Source: CAD feature listing. Evaluate the final solid. Frame: model axes, mm. A direction names the side the tool comes from. Coordinates: 2 decimals unless noted, no trailing zeros. Order: outer loops, then holes, each group sorted by start corner. A loop starts at its lowest first (then second) coordinate and runs counter-clockwise, first axis right, second up. Notation, with made-up numbers: (-38, 0.25) -> (4, 0.25) arc R26 cw to (4, 19.25) -> close; hole circle Ø11 at (13.5, 19). An arc over 180 degrees is marked (long way). Put each result on its own line as item: value.
Autodesk Inventor part; units mm, degrees
ref_plane "Start Plane" through (0, 0, 0) normal (0, 0, 1) x (1, 0, 0)
ref_plane "End Plane" through (0, 0, 300) normal (0, 0, 1) x (1, 0, 0)
ref_plane "Work Plane4" through (0, 12.7, 0) normal (0.7071, 0, -0.7071) x (-0.7071, 0, -0.7071)
ref_plane "Start Plane" through (0, 0, 0) normal (0, 0, 1) x (1, 0, 0)
ref_plane "End Plane" through (0, 0, 300) normal (0, 0, 1) x (1, 0, 0)
sketch "Sketch" plane through (0, 0, 0) normal (0, 0, 1) x (1, 0, 0)
  line L0 (25.4, 0) -> (0, 0)
  line L1 (0, 0) -> (0, 25.4)
  line L2 (0, 25.4) -> (1.651, 25.4)
  line L3 (3.175, 23.876) -> (3.175, 6.477)
  line L4 (6.477, 3.175) -> (23.876, 3.175)
  line L5 (25.4, 1.651) -> (25.4, 0)
  line L6 (0, -11.0414) -> (0, 31.5385) construction
  line L7 (-11.0414, 0) -> (31.5385, 0) construction
  arc A0 (3.175, 6.477) -> (6.477, 3.175) centre (6.477, 6.477) ccw
  arc A1 (3.175, 23.876) -> (1.651, 25.4) centre (1.651, 23.876) ccw
  arc A2 (25.4, 1.651) -> (23.876, 3.175) centre (23.876, 1.651) ccw
  line L8 (0, 40.0545) -> (0, -19.5574) construction
  line L9 (-19.5574, 0) -> (40.0545, 0) construction
  point P0 (3.175, 25.4)
  point P1 (3.175, 3.175)
  point P2 (25.4, 3.175)
  dimension "d0" = 25.4
  dimension "d1" = 25.4
  dimension "d2" = 3.175
  dimension "d3" = 3.175
  dimension "d10" = 0
  dimension "d11" = 0
  dimension "d14" = 3.302
  dimension "d15" = 1.524
extrude "Body" add sketch "Sketch" along normal up to surface (300 mm away) from surface at 0
sketch "Sketch3" plane through (0, 0, 0) normal (0, 0, 1) x (1, 0, 0)
  line L0 (0, 0) -> (10, 0)
ref_plane "Work Plane3" through (0, 0, 0) normal (0, -1, 0) x (1, 0, 0)
ref_plane "Work Plane4" through (0, 12.7, 0) normal (0.7071, 0, -0.7071) x (-0.7071, 0, -0.7071)
split "Split1" plane through (0, 12.7, 0) removes the side toward (0.7071, 0, -0.7071)
ref_plane "Work Plane5" through (0, 12.7, 300) normal (0.7071, 0, 0.7071) x (0.7071, 0, -0.7071)
split "Split2" plane through (0, 12.7, 300) removes the side toward (0.7071, 0, 0.7071)
sketch "Sketch4" plane through (0, 0, 0) normal (0, -1, 0) x (1, 0, 0)
  line L0 (-2, 0) -> (12, 0)
  line L1 (-2, 300) -> (12, 300)
  dimension "d17" = 300
equation "\"d0\" = G_H"
equation "\"d1\" = G_H"
equation "\"d2\" = G_T"
equation "\"d3\" = G_T"
equation "\"d14\" = G_IR"
equation "\"d15\" = G_ER"
equation "\"d4\" = G_L"
equation "\"G_H\" = 25.4"
equation "\"G_T\" = 3.175"
equation "\"G_ER\" = 1.524"
equation "\"G_IR\" = 3.302"
equation "\"G_L\" = d17"
equation "\"ex\" = 0"
equation "\"G_OFFSET_START\" = 0"
equation "\"G_OFFSET_END\" = 0"
equation "\"d13\" = G_OFFSET_END + B_L"
equation "\"B_L\" = 300"
properties part number "AISC - L 1 x 1 x 1/8 - 11.811" material "Steel, Mild"
1. Ray query, line 1 along Y through (x, z) = (7.25, 109.5) (3 decimals); line 2 along Y through (x, z) = (4.75, 117). Return the intervals inside material, ascending.
Numbers:
line 1: y = 0 to 3.175
line 2: y = 0 to 3.66
2. Cut plane C-C on y = 13.75. Output: boundary loops of the cut face in (x, z) (3 decimals), plus the area to 3 significant figures.
Numbers:
outline: (0, 0) -> (3.175, 3.175) -> (3.175, 296.825) -> (0, 300) -> close
area: 942 mm2
3. Set-up query: faces 4 (the flat face through (8, 2, 292)), 5 (the flat face through (3.175, 15, 148)). Return all of +Z, -Z, +X, -X, +Y, -Y with unobstructed straight access to the full face (end or side cutting, diameter ignored); none if empty.
Numbers:
face 4: +Z, +X, +Y, -Y
face 5: +Z, -Z, +X, +Y
4. Pull-direction query (X, two-part tool) for faces 1 (the flat face through (0, 13, 148)), 2 (the flat face through (13, 0, 148)), 3 (the flat face through (8, 2, 8)); classes: pulls with the +X half, pulls with the -X half, needs draft (parallel to the pull), parting line crosses it, or undercut.
Numbers:
face 1: pulls with the -X half
face 2: needs draft
face 3: pulls with the +X half
5. First-contact query: pin 1 (4 mm diameter, centred on y = 18.5, z = 32.5, fed in from -X); pin 2 (5 mm diameter, centred on x = 13, z = 90, fed in from +Y) (3 decimals); pin 3 (6 mm diameter, centred on y = 16.5, z = 97, fed in from +X) (3 decimals); pin 4 (6 mm diameter, centred on x = 19.5, y = 4, fed in from -Z). Flat tips, straight axial feed; report the tip coordinate or a pass-through.
Numbers:
pin 1: stops at x = 0
pin 2: stops at y = 3.175
pin 3: stops at x = 3.175
pin 4: stops at z = 16.62
6. Cut plane A-A on z = 235. Output: boundary loops of the cut face in (x, y) (3 decimals), plus the area to 3 significant figures.
Numbers:
outline: (0, 0) -> (25.4, 0) -> (25.4, 1.651) arc R1.524 ccw to (23.876, 3.175) -> (6.477, 3.175) arc R3.302 cw to (3.175, 6.477) -> (3.175, 23.876) arc R1.524 ccw to (1.651, 25.4) -> (0, 25.4) -> close
area: 153 mm2
7. Cut plane B-B on x = 13. Output: boundary loops of the cut face in (y, z) (3 decimals).
Numbers:
outline: (0, 13) -> (3.175, 13) -> (3.175, 287) -> (0, 287) -> close
